from build123d import *

# Parameters (mm, degrees)
F0_W     = 36
F0_H     = 165
F1_DEPTH = 12
F3_D     = 6.3
F3_DEPTH = 40
F3_TIP   = 1.8927109499
F5_D     = 4.2
F5_DEPTH = 4
F5_TIP   = 1.2618073


with BuildPart() as f1:
    # F0 (on Top) → F1 (new body)
    with BuildSketch(Plane.XY):
        Rectangle(F0_W, F0_H)
    extrude(amount=F1_DEPTH)

    # F3
    with Locations(Plane.XY.offset(12)):
        with Locations((-0.5, -66.5), (12, 9), (12, 69)):
            Hole(F3_D / 2, depth=F3_DEPTH)
            with Locations((0, 0, -(F3_DEPTH + F3_TIP / 2))):  # 118° drill point
                Cone(0, F3_D / 2, F3_TIP, mode=Mode.SUBTRACT)

    # F5
    with Locations(Plane.YZ.offset(18)):
        with Locations((26.5, 6), (54.5, 6)):
            Hole(F5_D / 2, depth=F5_DEPTH)
            with Locations((0, 0, -(F5_DEPTH + F5_TIP / 2))):  # 118° drill point
                Cone(0, F5_D / 2, F5_TIP, mode=Mode.SUBTRACT)


solid = f1.part
CAD build for the part. Positions are in the model's coordinates, mm. A direction names the side the tool comes from. Give positions to 0.01 mm unless a question says otherwise; leave off trailing zeros. Write each loop counter-clockwise with the first axis right and the second up, starting at its lowest first coordinate (ties: lowest second). Pieces come first, ordered by that corner, then holes. Notation, with made-up numbers: M -38.5,31 L 6.5,31 A21 ccw 6.5,70 Z; hole C 66,38.5 d3. An arc over 180 degrees is marked long. Put each result on its own line as item: value. Start each with the question number.
(1) Probe L1, parallel to Y at x = 12, z = 5; L2, parallel to Y at x = 15.9, z = 6; L3, parallel to Y at x = -0.5, z = 2.5. List the from-to ranges inside material, lowest first.
(2) Flat gauge pins, fed straight in: pin 1 Ø2.5 at (y, z) = (26.5, 6) entering from +X; pin 2 Ø5 at (x, y) = (12, 9) entering from +Z. Where does each tip first touch, or does it go through?
(3) Which spindle directions (+Z, -Z, +X, -X, +Y, -Y) get a long thin tool onto all of the face, cutting with end or side? Do faces 4 (the face through (15.972, 52.497, 6.631)), 5 (the face through (0, -82.5, 6)). Say none if no direction does.
(4) Mould opens along X. For faces 1 (the face through (18, -1, 6)), 2 (the face through (0, 82.5, 6)), 3 (the face through (14.5, 67.083, 5.916)) say: +X half, -X half, draft (parallel to the pull), parting line (faces both ways), or undercut.
(5) Band-saw the part on C-C, the plane z = 2.5. Write the cut outline in (x, y).
(6) Band-saw the part on B-B, the plane y = 69. Write the cut outline in (x, z), and give its area (3 significant figures).
(7) Band-saw the part on A-A, the plane x = -0.5. Write the cut outline in (y, z), and give its area (3 significant figures).
Response values:
1. L1: y = -82.5 to 5.85, 12.15 to 65.85, 72.15 to 82.5
1. L2: y = -82.5 to 24.4, 28.6 to 52.4, 56.6 to 82.5
1. L3: y = -82.5 to -69.65, -63.35 to 82.5
2. pin 1: stops at x = 13.49
2. pin 2: passes through
3. face 4: +X
3. face 5: +Z, -Z, +X, -X, -Y
4. face 1: +X half
4. face 2: draft
4. face 3: undercut
5. outline: M -18,-82.5 L 18,-82.5 L 18,82.5 L -18,82.5 Z; hole C -0.5,-66.5 d6.3; hole C 12,9 d6.3; hole C 12,69 d6.3
6. outline: M -18,0 L 8.85,0 L 8.85,12 L -18,12 Z; M 15.15,0 L 18,0 L 18,12 L 15.15,12 Z
6. area: 356 mm2
7. outline: M -82.5,0 L -69.65,0 L -69.65,12 L -82.5,12 Z; M -63.35,0 L 82.5,0 L 82.5,12 L -63.35,12 Z
7. area: 1,900 mm2
